CAD build for the part. Positions are in the model's coordinates, mm. Face numbers are marked on the shaded views. A direction names the side the tool comes from. Round coordinates to 2 decimals unless told otherwise and drop trailing zeros. Loops run counter-clockwise (first coordinate to the right, second up) from the corner with the lowest first, then second, coordinate; pieces in that order, holes last. Notation, with made-up numbers: (19.5, 87) -> (61.5, 87) arc R24 cw to (61.5, 126) -> close; hole circle Ø8 at (-21, 68). An arc over 180 degrees is marked (long way). Answer as CSV lines item,"result".
```python
from build123d import *

# Parameters (mm, degrees)
F1_DEPTH = 5.08
F2_R     = 1.651
F4_D     = 3.3


with BuildPart() as f1:
    # F0 (on Front) → F1 (new body)
    with BuildSketch(Plane.XZ):
        with BuildLine():
            Line((-26.6248177087, 44.2240222495), (-26.6248177087, 37.1401777957))
            Line((-26.6248177087, 37.1401777957), (-26.6248177087, 15.790813717))
            Line((-26.6248177087, 15.790813717), (-18.0322819572, 15.790813717))
            Line((-18.0322819572, 15.790813717), (-9.4473101199, 15.790813717))
            Line((-9.4473101199, 15.790813717), (-9.4473101199, 23.6617988805))
            Line((-9.4473101199, 23.6617988805), (-16.3273841628, 23.6617988805))
            add(Edge.make_bspline(
                [(-16.3273841628, 23.6617988805), (-16.2021531976, 23.1573319897), (-16.1372444387, 22.7565283285), (-16.1473177087, 22.4913693964)],
                knots=[0.9536770063, 0.9536770063, 0.9536770063, 0.9536770063, 1, 1, 1, 1], degree=3))
            add(Edge.make_bspline(
                [(-16.1473177087, 22.4913693964), (-16.1800367938, 21.6301041251), (-17.0038324761, 22.1999200382), (-18.0322819572, 23.6617988805)],
                knots=[0, 0, 0, 0, 0.1504621604, 0.1504621604, 0.1504621604, 0.1504621604], degree=3))
            add(Edge.make_bspline(
                [(-18.0322819572, 23.6617988805), (-18.4185584968, 24.2108676593), (-20.6372456091, 27.8178237541), (-22.7930713687, 34.2033705284), (-23.4498177087, 37.1401777957)],
                knots=[0.1504621604, 0.1504621604, 0.1504621604, 0.1504621604, 0.2069744186, 0.4524830891, 0.4524830891, 0.4524830891, 0.4524830891], degree=3))
            add(Edge.make_bspline(
                [(-23.4498177087, 37.1401777957), (-23.7877118735, 38.6511569639), (-23.8355675171, 39.5655078846), (-23.4498177087, 39.3262133002)],
                knots=[0.4524830891, 0.4524830891, 0.4524830891, 0.4524830891, 0.578796617, 0.578796617, 0.578796617, 0.578796617], degree=3))
            Line((-23.4498177087, 39.3262133002), (-23.4498177087, 44.2240222495))
            Line((-23.4498177087, 44.2240222495), (-23.4498177087, 49.9301888049))
            ThreePointArc((-23.4498177087, 49.9301888049), (-25.0373177087, 51.5176888049), (-26.6248177087, 49.9301888049))
            Line((-26.6248177087, 49.9301888049), (-26.6248177087, 44.2240222495))
        make_face()
        with BuildLine():
            Line((-23.4498177087, 37.1401777957), (-23.4498177087, 39.3262133002))
            add(Edge.make_bspline(
                [(-23.4498177087, 37.1401777957), (-23.7877118735, 38.6511569639), (-23.8355675171, 39.5655078846), (-23.4498177087, 39.3262133002)],
                knots=[0.4524830891, 0.4524830891, 0.4524830891, 0.4524830891, 0.578796617, 0.578796617, 0.578796617, 0.578796617], degree=3))
        make_face()
        with BuildLine():
            add(Edge.make_bspline(
                [(-16.3273841628, 23.6617988805), (-16.2021531976, 23.1573319897), (-16.1372444387, 22.7565283285), (-16.1473177087, 22.4913693964)],
                knots=[0.9536770063, 0.9536770063, 0.9536770063, 0.9536770063, 1, 1, 1, 1], degree=3))
            Line((-16.3273841628, 23.6617988805), (-18.0322819572, 23.6617988805))
            add(Edge.make_bspline(
                [(-16.1473177087, 22.4913693964), (-16.1800367938, 21.6301041251), (-17.0038324761, 22.1999200382), (-18.0322819572, 23.6617988805)],
                knots=[0, 0, 0, 0, 0.1504621604, 0.1504621604, 0.1504621604, 0.1504621604], degree=3))
        make_face()
    extrude(amount=F1_DEPTH)

    # F2
    f2_edges = [f1.edges().sort_by_distance(p)[0] for p in [
        (-18.036064, -5.08, 15.790814),
        (-18.036064, 0, 15.790814),
    ]]
    fillet(f2_edges, radius=F2_R)

    # F4 (through all)
    with Locations(Plane(origin=(-26.6248177087, 0, 0), x_dir=(0, -1, 0), z_dir=(-1, 0, 0))):
        with Locations((2.54, 47.7136392146), (2.54, 19.4669695918)):
            Hole(F4_D / 2)


solid = f1.part
```
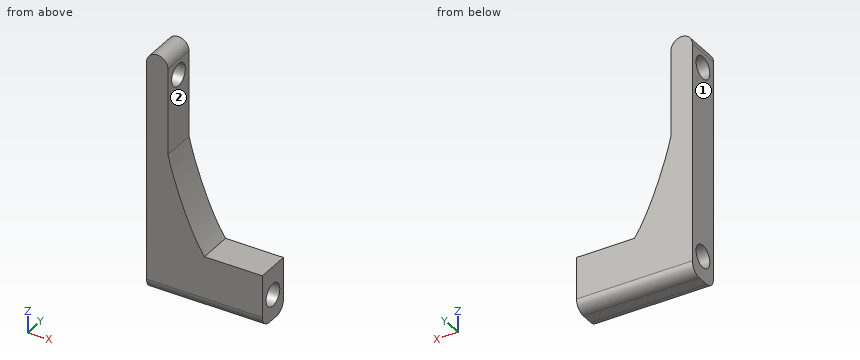
Q1. Drop flat-ended pins along their axis: pin 1 Ø3 at (y, z) = (-2.54, 19.47) entering from +X; pin 2 Ø2.5 at (x, y) = (-12.5, -2) entering from +Z. Give the stop position or say it passes through.
Results:
pin 1,"through"
pin 2,"z = 23.66"
Q2. Slice it at B-B, the plane y = -2.54. Count the separate pieces of the cut face and the enclosed holes in it, and give its area (3 significant figures).
Results:
separate pieces,"3"
enclosed holes,"0"
area,"186 mm2"
Q3. Slice it at A-A, the plane x = -24. Give the cut face in (y, z), and give its area (3 significant figures).
Results:
outline,"(-5.08, 17.44) arc R1.65 ccw to (-3.43, 15.79) -> (-1.65, 15.79) arc R1.65 ccw to (0, 17.44) -> (0, 51.13) -> (-5.08, 51.13) -> close; hole circle Ø3.3 at (-2.54, 19.47); hole circle Ø3.3 at (-2.54, 47.71)"
area,"161 mm2"
Q4. Slice it at C-C, the plane x = -17. Give the cut face in (y, z), and give its area (3 significant figures).
Results:
outline,"(-5.08, 17.44) arc R1.65 ccw to (-3.43, 15.79) -> (-1.65, 15.79) arc R1.65 ccw to (0, 17.44) -> (0, 23.66) -> (-5.08, 23.66) -> close; hole circle Ø3.3 at (-2.54, 19.47)"
area,"30.3 mm2"
Q5. Tool access for the marked faces 1 and 2: list every direction of +Z, -Z, +X, -X, +Y, -Y with a clear straight run to the whole face (end or side of a thin tool).
Results:
face 1,"+Z, -Z, -X, +Y, -Y"
face 2,"+Z, +X, +Y, -Y"
Q6. Slice it at D-D, the plane z = 42.5. Give the cut face in (x, y), and give its area (3 significant figures).
Results:
outline,"(-26.62, -5.08) -> (-23.45, -5.08) -> (-23.45, 0) -> (-26.62, 0) -> close"
area,"16.1 mm2"
Q7. Probe L1, parallel to Z at x = -14.25, y = -2.45; L2, parallel to X at y = -2.15, z = 42.5; L3, parallel to Z at x = -10.25, y = -1.8. List the from-to ranges inside material, lowest first. Write a range as [from, to].
Results:
L1,"[15.79, 17.82], [21.11, 23.66]"
L2,"[-26.62, -23.45]"
L3,"[15.79, 17.99], [20.94, 23.66]"
